from build123d import *

# Parameters (mm, degrees)
BOSS_EXTRUDE1_DEPTH = 30
BOSS_EXTRUDE2_START = 2.175
SKETCH2_R           = 1.55
BOSS_EXTRUDE2_DEPTH = 5


with BuildPart() as part:
    # Sketch1 → Boss-Extrude1 (new, symmetric)
    with BuildSketch(Plane.XY):
        Polygon((-26.5, 1), (-26.5, 0), (26.5, 0), (26.5, 1), (24.5, 1), (24.5, 3), (30, 3), (30, 24), (-30, 24), (-30, 3), (-24.5, 3), (-24.5, 1), align=None)
    extrude(amount=BOSS_EXTRUDE1_DEPTH, both=True)

    # Sketch2 → Boss-Extrude2 (add)
    with BuildSketch(Plane(origin=(0, 0, 0), x_dir=(0, 0, -1), z_dir=(1, 0, 0)).offset(BOSS_EXTRUDE2_START)):
        with BuildLine():
            ThreePointArc((36.015485064, 2.124014936), (37.798326563, 3.786794145), (37.793319851, 6.224689434))
            Line((37.793319851, 6.224689434), (30, 24))
            Line((30, 24), (30, 0))
            Line((30, 0), (36.015485064, 2.124014936))
        make_face()
        with Locations((35, 5)):
            Circle(SKETCH2_R, mode=Mode.SUBTRACT)
    extrude(amount=BOSS_EXTRUDE2_DEPTH)


solid = part.part
Design review of the part built by this model. Coordinates are the model's own, in mm. A direction names the side the tool comes from. Give positions to 0.01 mm unless a question says otherwise; leave off trailing zeros. Write each loop counter-clockwise with the first axis right and the second up, starting at its lowest first coordinate (ties: lowest second). Pieces come first, ordered by that corner, then holes. Notation, with made-up numbers: M 73,79 L 77,79 A23 cw 77,100 Z; hole C -19,70.5 d8. An arc over 180 degrees is marked long. Answer as a JSON object with one key per item and string values. Group by question number.
1) We need section B-B (z = -35). Give the boundary of the cut face in (x, y) (3 decimals).
2) We need section C-C (z = 22.5). Give the boundary of the cut face in (x, y), and give its area (3 significant figures).
3) For line 1 along Z through (x, y) = (21.5, 6.25); line 2 along X through (y, z) = (18.75, -31) (3 decimals); line 3 along Y through (x, z) = (5.8, -35), list the stretches that pass through material, from the lowest coordinate up.
4) We need section D-D (y = 18). Give the boundary of the cut face in (x, z) (3 decimals).
5) Tool access review of faces 1 (the face through (-27, 3, 0)), 2 (the face through (24.5, 2, 0)), 3 (the face through (7.175, 10, -33)), 4 (the face through (4.64, 5.466, -36.478)), 5 (the face through (2.175, 10, -33)): name each direction out of +Z, -Z, +X, -X, +Y, -Y from which nothing blocks a thin tool from reaching the whole face with its end or side.
6) Mouldability with a two-part tool opening along Y and no side actions: class faces 6 (the face through (27, 3, 0)), 7 (the face through (4.64, 14.99, -33.95)), 8 (the face through (18, 12, -30)) as released by +Y, released by -Y, zero draft, split by the parting line, or undercut.
7) Clearance check with flat-ended pins moving along their axes: pin 1 Ø1.5 at (x, z) = (7, -22.5) entering from -Y; pin 2 Ø0.5 at (y, z) = (0.5, 4) entering from -X; pin 3 Ø7 at (x, y) = (21.5, 11.5) entering from -Z; pin 4 Ø1.6 at (y, z) = (2, 2.5) entering from +X. State where each tip first meets the part, or that it passes through.
8) We need section A-A (y = 5). Give the boundary of the cut face in (x, z) (3 decimals), and give its area (3 significant figures).
Answer key:
{
 "1": {"outline": "M 2.175,1.765 L 7.175,1.765 L 7.175,3.45 L 2.175,3.45 Z; M 2.175,6.55 L 7.175,6.55 L 7.175,12.596 L 2.175,12.596 Z"},
 "2": {"outline": "M -30,3 L -24.5,3 L -24.5,1 L -26.5,1 L -26.5,0 L 26.5,0 L 26.5,1 L 24.5,1 L 24.5,3 L 30,3 L 30,24 L -30,24 Z", "area": "1,410 mm²"},
 "3": {"line 1": "z = -30 to 30", "line 2": "x = 2.175 to 7.175", "line 3": "y = 1.77 to 3.45, 6.55 to 12.6"},
 "4": {"outline": "M -30,-30 L 2.175,-30 L 2.175,-32.631 L 7.175,-32.631 L 7.175,-30 L 30,-30 L 30,30 L -30,30 Z"},
 "5": {"face 1": "+Z, -Z, -X", "face 2": "+Z, -Z, +X", "face 3": "-Z, +X, +Y, -Y", "face 4": "+X, -X", "face 5": "-Z, -X, +Y, -Y"},
 "6": {"face 6": "undercut", "face 7": "released by +Y", "face 8": "zero draft"},
 "7": {"pin 1": "stops at y = 0", "pin 2": "stops at x = -26.5", "pin 3": "stops at z = -30", "pin 4": "stops at x = 24.5"},
 "8": {"outline": "M -30,-30 L 2.175,-30 L 2.175,-33.45 L 7.175,-33.45 L 7.175,-30 L 30,-30 L 30,30 L -30,30 Z; M 2.175,-38.05 L 7.175,-38.05 L 7.175,-36.55 L 2.175,-36.55 Z", "area": "3,620 mm²"}
}
